Work out the finished part from the listing and answer in its coordinate system (mm). A direction names the side the tool comes from. Coordinates: 2 decimals unless noted, no trailing zeros. Order: outer loops, then holes, each group sorted by start corner. A loop starts at its lowest first (then second) coordinate and runs counter-clockwise, first axis right, second up.
1. The part is cut by section D-D, the plane y = -15. Give the vertices of the cut face in (x, z).
2. Determine the mould class of faces 6 (the flat face through (0, -3, 23)), 7 (the cylindrical face through (35.76, -2.96, 44.08)), 8 (the flat face through (21, -29, 3)) for opening direction X: +X half, -X half, draft (parallel to the pull), parting line (faces both ways), or undercut.
3. The part is cut by section C-C, the plane y = -7.5. Give the vertices of the cut face in (x, z).
4. Find the intervals of material crossed by probe 1 along Z at (x, y) = (36.5, -3.65); probe 2 along Z at (x, y) = (36.5, -0.7); probe 3 along X at (y, z) = (-13.6, 1.7), in increasing order.
5. A tool of negligible diameter and unlimited length cuts with its end or side. For faces 1 (the flat face through (21, -11, 15.2)), 2 (the flat face through (38, -3, 13)), 3 (the flat face through (42, -21, 2)), 4 (the flat face through (21, -16, 18)), 5 (the flat face through (33.5, -11, 18)), from which of +Z, -Z, +X, -X, +Y, -Y can it reach the whole face along a straight path? Write none if from no direction.
6. Flat-ended cylindrical pins translate along their axes: pin 1 Ø8 at (x, z) = (32.5, 32.5) entering from -Y; pin 2 Ø5.5 at (y, z) = (-22.5, 3) entering from +X; pin 3 Ø5 at (x, y) = (31.5, -10) entering from +Z; pin 4 Ø2.5 at (x, z) = (5.5, 14.5) entering from +Y. Find the tip coordinate at first contact, or state that the pin passes through.
7. The part is cut by section B-B, the plane z = 14.5. Give the vertices of the cut face in (x, y).
8. The part is cut by section A-A, the plane x = 21. Give the vertices of the cut face in (y, z), then the cut area to 3 significant figures.
```python
from build123d import *

# Parameters (mm, degrees)
F0_W      = 42
F0_H      = 51
F0_R      = 11.1
F1_DEPTH  = 6
F2_SIZE   = 4
F3_W      = 42
F3_H      = 5
F4_DEPTH  = 23
F6_DEPTH  = 10
F7_R      = 1.6
F8_DEPTH  = 25
F9_R      = 2.5
F10_DEPTH = 6
F11_R     = 3
F12_DEPTH = 3
F14_DEPTH = 5
F15_R     = 5


with BuildPart() as f1:
    # F0 (on Front) → F1 (new body)
    with BuildSketch(Plane.XZ):
        with Locations((21, 25.5)):
            Rectangle(F0_W, F0_H)
        with Locations((21, 30)):
            Circle(F0_R, mode=Mode.SUBTRACT)
    extrude(amount=F1_DEPTH)

    # F2
    f2_edges = [f1.edges().sort_by_distance(p)[0] for p in [
        (0, -3, 51),
        (42, -3, 51),
    ]]
    chamfer(f2_edges, length=F2_SIZE)

    # F3 (on face) → F4 (join)
    with BuildSketch(Plane.XZ.offset(6)):
        with Locations((21, 2.5)):
            Rectangle(F3_W, F3_H)
    extrude(amount=F4_DEPTH)

    # F5 (on face) → F6 (join)
    with BuildSketch(Plane.XZ.offset(6)):
        with BuildLine():
            Line((14.2346470898, 21.2), (8.5, 21.2))
            Line((8.5, 21.2), (8.5, 15.2))
            Line((8.5, 15.2), (33.5, 15.2))
            Line((33.5, 15.2), (33.5, 21.2))
            Line((33.5, 21.2), (27.7653529102, 21.2))
            ThreePointArc((27.7653529102, 21.2), (21, 18.9), (14.2346470898, 21.2))
        make_face()
    extrude(amount=F6_DEPTH)

    # F7 (on face) → F8 (cut)
    with BuildSketch(Plane(origin=(0, 0, 0), x_dir=(-1, 0, 0), z_dir=(0, 1, 0))):
        with Locations((-36.5, 45.5)):
            Circle(F7_R)
        with Locations((-5.5, 45.5)):
            Circle(F7_R)
        with Locations((-5.5, 14.5)):
            Circle(F7_R)
        with Locations((-36.5, 14.5)):
            Circle(F7_R)
    extrude(amount=-F8_DEPTH, mode=Mode.SUBTRACT)

    # F9 (on Top) → F10 (cut)
    with BuildSketch(Plane.XY):
        with Locations((3.1, -13.6)):
            Circle(F9_R)
        with Locations((38.9, -13.6)):
            Circle(F9_R)
    extrude(amount=F10_DEPTH, mode=Mode.SUBTRACT)

    # F11 (on face) → F12 (cut)
    with BuildSketch(Plane.XZ.offset(6)):
        with Locations((5.5, 14.5)):
            Circle(F11_R)
        with Locations((36.5, 14.5)):
            Circle(F11_R)
    extrude(amount=-F12_DEPTH, mode=Mode.SUBTRACT)

    # F13 (on face) → F14 (join)
    with BuildSketch(Plane.XY.offset(5)):
        with BuildLine():
            Line((0, -18.7371198156), (0, -8.4628801844))
            ThreePointArc((0, -8.4628801844), (-2.9, -13.6), (0, -18.7371198156))
        make_face()
        with BuildLine():
            ThreePointArc((44.9, -13.6), (44.124940191, -10.6504237592), (42, -8.4628801844))
            Line((42, -8.4628801844), (42, -18.7371198156))
            ThreePointArc((42, -18.7371198156), (44.124940191, -16.5495762408), (44.9, -13.6))
        make_face()
    extrude(amount=-F14_DEPTH)

    # F15
    f15_edges = [f1.edges().sort_by_distance(p)[0] for p in [
        (0, -29, 2.5),
        (42, -29, 2.5),
    ]]
    fillet(f15_edges, radius=F15_R)


solid = f1.part
```
Geometry says:
1. outline: (-2.73, 0) - (1.03, 0) - (1.03, 5) - (-2.73, 5) - close; (5.17, 0) - (36.83, 0) - (36.83, 5) - (5.17, 5) - close; (8.5, 15.2) - (33.5, 15.2) - (33.5, 21.2) - (27.77, 21.2) arc R11.1 cw to (14.23, 21.2) - (8.5, 21.2) - close; (40.97, 0) - (44.73, 0) - (44.73, 5) - (40.97, 5) - close
2. face 6: -X half
2. face 7: undercut
2. face 8: draft
3. outline: (0, 0) - (42, 0) - (42, 5) - (0, 5) - close; (8.5, 15.2) - (33.5, 15.2) - (33.5, 21.2) - (27.77, 21.2) arc R11.1 cw to (14.23, 21.2) - (8.5, 21.2) - close
4. probe 1: z = 0 to 11.5, 17.5 to 43.9, 47.1 to 51
4. probe 2: z = 0 to 12.9, 16.1 to 43.9, 47.1 to 51
4. probe 3: x = -2.9 to 0.6, 5.6 to 36.4, 41.4 to 44.9
5. face 1: +X, -X, -Y
5. face 2: -Y
5. face 3: +Z, -Z, +X, -Y
5. face 4: +Z, +X, -X, -Y
5. face 5: +Z, +X, -Y
6. pin 1: stops at y = -6
6. pin 2: stops at x = 42
6. pin 3: stops at z = 21.2
6. pin 4: passes through
7. outline: (0, -6) - (2.5, -6) - (2.5, -3) - (3.9, -3) - (3.9, 0) - (0, 0) - close; (7.1, -3) - (8.5, -3) - (8.5, -6) - (33.5, -6) - (33.5, -3) - (34.9, -3) - (34.9, 0) - (7.1, 0) - close; (38.1, -3) - (39.5, -3) - (39.5, -6) - (42, -6) - (42, 0) - (38.1, 0) - close
8. outline: (-29, 0) - (0, 0) - (0, 18.9) - (-16, 18.9) - (-16, 15.2) - (-6, 15.2) - (-6, 5) - (-29, 5) - close; (-6, 41.1) - (0, 41.1) - (0, 51) - (-6, 51) - close
8. area: 325 mm2
